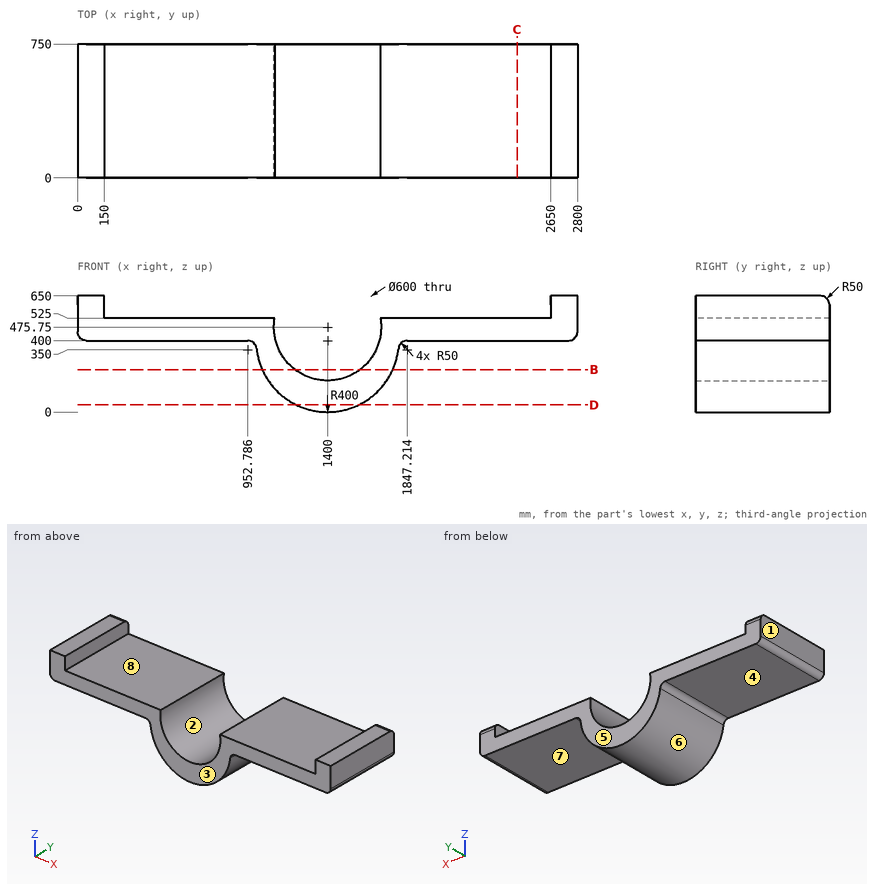
Geometry check sheet. Reference: drawing and pictorial views, mm from the part's lowest x, y, z. A direction names the side the tool comes from. Give positions to 0.01 mm unless a question says otherwise; leave off trailing zeros. Loops run counter-clockwise (first coordinate to the right, second up) from the corner with the lowest first, then second, coordinate; pieces in that order, holes last. Notation, with made-up numbers: M -20.5,48.25 L -8.5,48.25 A27 cw -8.5,65.25 Z; hole C 11,85 d3. An arc over 180 degrees is marked long. Use a Markdown table: item, result. Add a question column.
Q1. Sectioned sample at C-C, the plane x = 2462. Record the cut outline in (y, z).
Q2. Go/stop test with flat-tipped pins: pin 1 (12 mm diameter, centred on y = 510, z = 209, fed in from -X); pin 2 (6 mm diameter, centred on y = 127.5, z = 173, fed in from +X); pin 3 (10 mm diameter, centred on x = 1425.5, y = 464.5, fed in from -Z). Record where each tip stops, or that it passes through.
Q3. Mould release check, pull along X, two halves, no side actions. Record for the marked faces 1, 2 and 3: pulls with the +X half, pulls with the -X half, needs draft (parallel to the pull), parting line crosses it, or undercut.
Q4. Scan lines: line 1 along X through (y, z) = (50.5, 564.5); line 2 along Z through (x, y) = (318, 662); line 3 along X through (y, z) = (695.5, 200.5) (1 decimal). Record each from-to range of solid material in increasing order. Write a range as [from, to].
Q5. Sectioned sample at D-D, the plane z = 40. Record the cut outline in (x, y), then the cut area to 3 significant figures.
Q6. Sectioned sample at B-B, the plane z = 238. Record the cut outline in (x, y), then the cut area to 3 significant figures.
Q7. Tool access check on the marked faces 4, 5, 6, 7 and 8. Record the directions out of +Z, -Z, +X, -X, +Y, -Y that give a thin tool (end or side, any length) a straight path to the whole face; none if there is none.
Verdict:
| question | item | result |
|---|---|---|
| 1 | outline | M 0,400 L 750,400 L 750,525 L 0,525 Z |
| 2 | pin 1 | x = 1045.35 |
| 2 | pin 2 | x = 1731.4 |
| 2 | pin 3 | z = 0.53 |
| 3 | face 1 | pulls with the -X half |
| 3 | face 2 | undercut |
| 3 | face 3 | needs draft |
| 4 | line 1 | [0, 150], [2650, 2800] |
| 4 | line 2 | [400, 525] |
| 4 | line 3 | [1053.3, 1280.7], [1519.3, 1746.7] |
| 5 | outline | M 1225.64,0 L 1574.36,0 L 1574.36,750 L 1225.64,750 Z |
| 5 | area | 262,000 mm^2 |
| 6 | outline | M 1034.27,0 L 1217.04,0 L 1217.04,750 L 1034.27,750 Z; M 1582.96,0 L 1765.73,0 L 1765.73,750 L 1582.96,750 Z |
| 6 | area | 274,000 mm^2 |
| 7 | face 4 | -Z, -X, +Y, -Y |
| 7 | face 5 | +Z, -Z, +X, -X, +Y |
| 7 | face 6 | -Z, +Y, -Y |
| 7 | face 7 | -Z, +X, +Y, -Y |
| 7 | face 8 | +Z, +Y, -Y |
